Part model, mm, in its own coordinate system. Round coordinates to 2 decimals unless told otherwise and drop trailing zeros. Write each loop counter-clockwise with the first axis right and the second up, starting at its lowest first coordinate (ties: lowest second). Pieces come first, ordered by that corner, then holes. Notation, with made-up numbers: (-12.5, 1) -> (35.5, 1) arc R17 ccw to (35.5, 6) -> close; hole circle Ø3 at (33.25, -13). An arc over 180 degrees is marked (long way). Return JSON: item names as keys, results as strings. Group by question number.
(1) Saw through at A-A (z = -1.1). List the corners of the cut face in (x, y).
(2) Mould opens along X. For faces 1 (the flat face through (2, 3, 0)), 2 (the flat face through (-6.35, 0, -2)), 3 (the cylindrical face through (2.435, 0.767, -2.402)) say: +X half, -X half, draft (parallel to the pull), parting line (faces both ways), or undercut.
(3) Drill centre lines: L1, parallel to X at y = 2.25, z = -1.05; L2, parallel to Y at x = 5, z = -1.6; L3, parallel to Y at x = -4, z = -2.75. Where is each one in solid material? Low to high. Write a range as from..to.
(4) Drop flat-ended pins along their axis: pin 1 Ø4 at (x, y) = (-0.5, 2.5) entering from +Z; pin 2 Ø1.5 at (y, z) = (4.5, -3.5) entering from +X; pin 3 Ø1.5 at (x, y) = (0.5, 2) entering from +Z. Give the stop position or say it passes through.
from build123d import *

# Parameters (mm, degrees)
BASENUT_START = -4.7752
BASENUTSKE_R  = 2.5527
BASENUT_DEPTH = 4.7752


with BuildPart() as part:
    # BaseNutSke → BaseNut (new body)
    with BuildSketch(Plane.XY.offset(BASENUT_START)):
        Polygon((6.35, 3.666174209), (6.35, -3.666174209), (0, -7.332348419), (-6.35, -3.666174209), (-6.35, 3.666174209), (0, 7.332348419), align=None)
        Circle(BASENUTSKE_R, mode=Mode.SUBTRACT)
    extrude(amount=BASENUT_DEPTH)

    # Sketch3 → Double-Chamfer (revolve, cut)
    with BuildSketch(Plane(origin=(0, 0, 0), x_dir=(0, 0, -1), z_dir=(1, 0, 0))):
        Polygon((4.7752, 6.35), (4.1402, 7.332348419), (4.1402, 20.032348419), (17.4752, 20.032348419), (17.4752, 6.35), align=None)
        Polygon((0.635, 20.032348419), (-12.7, 20.032348419), (-12.7, 6.35), (0, 6.35), (0.635, 7.332348419), align=None)
    revolve(axis=Axis((0, 0, 0), (0, 0, -1)), mode=Mode.SUBTRACT)

    # EndChamferSke → EndChamfer (revolve, cut)
    with BuildSketch(Plane(origin=(0, 0, 0), x_dir=(0, 0, -1), z_dir=(1, 0, 0)), mode=Mode.PRIVATE) as endchamfer_sk:
        Polygon((4.7498, 3.175), (4.270486934, 2.49047), (4.8006, 2.49047), (4.8006, 3.175), align=None)
        Polygon((-0.0508, 3.175), (0, 3.175), (0.479313066, 2.49047), (-0.0508, 2.49047), align=None)
    revolve(endchamfer_sk.sketch.rotate(Axis((0, 0, -25.037505729), (0, 0, -1)), 90), axis=Axis((0, 0, -25.037505729), (0, 0, -1)), mode=Mode.SUBTRACT)


solid = part.part
Computed values:
{
 "1": {"outline": "(-6.35, -3.67) -> (0, -7.33) -> (6.35, -3.67) -> (6.35, 3.67) -> (0, 7.33) -> (-6.35, 3.67) -> close; hole circle Ø5.11 at (0, 0)"},
 "2": {"face 1": "draft", "face 2": "-X half", "face 3": "undercut"},
 "3": {"L1": "-6.35..-1.21, 1.21..6.35", "L2": "-4.45..4.45", "L3": "-5.02..5.02"},
 "4": {"pin 1": "z = 0", "pin 2": "x = 6.2", "pin 3": "z = -0.25"}
}
